Source: CAD feature listing. Evaluate the final solid. Frame: model axes, mm. Coordinates: 2 decimals unless noted, no trailing zeros. Write each loop counter-clockwise with the first axis right and the second up, starting at its lowest first coordinate (ties: lowest second). Pieces come first, ordered by that corner, then holes. Notation, with made-up numbers: M 66.25,42 L 125.25,42 A28 ccw 125.25,65 Z; hole C 27,34 d6. An arc over 180 degrees is marked long. Answer as CSV lines item,"result". Start each with the question number.
1. Line query: probe 1 along X at (y, z) = (8.5, -0.25); probe 2 along X at (y, z) = (-15, -0.4); probe 3 along X at (y, z) = (0, -0.25). Output: solid intervals per line, ascending. Write a range as [from, to].
2. Contact query for a flat-ended pin moving along its axis: pin 1 Ø3 at (x, y) = (26.5, -15) entering from +Z. Output: stop coordinate, or through.
3. Section C-C on y = 15. Return the cut outline in (x, z).
4. Section D-D on x = -4.25. Return the cut outline in (y, z).
5. Section A-A on y = 0. Return the cut outline in (x, z).
6. Section B-B on x = 26.5. Return the cut outline in (y, z), plus the area to 3 significant figures.
Autodesk Inventor part; units mm, degrees
ref_plane "YZ Plane" through (0, 0, 0) normal (1, 0, 0) x (0, 1, 0)
ref_plane "XZ Plane" through (0, 0, 0) normal (0, 1, 0) x (-1, 0, 0)
ref_plane "XY Plane" through (0, 0, 0) normal (0, 0, 1) x (1, 0, 0)
sketch "Sketch1" plane through (0, 0, 0) normal (0, 0, 1) x (1, 0, 0)
  line L0 (0, -42.5799) -> (0, 42.5799)
  line L1 (-42.5799, 0) -> (42.5799, 0)
  line L2 (-28, 30) -> (28, 30)
  line L3 (30, 28) -> (30, -28)
  line L4 (28, -30) -> (-28, -30)
  line L5 (-30, -28) -> (-30, 28)
  arc A0 (-28, 30) -> (-30, 28) centre (-28, 28) ccw
  arc A1 (30, 28) -> (28, 30) centre (28, 28) ccw
  arc A2 (28, -30) -> (30, -28) centre (28, -28) ccw
  arc A3 (-30, -28) -> (-28, -30) centre (-28, -28) ccw
  point P0 (0, 0)
  point P1 (-30, 30)
  point P2 (30, 30)
  point P3 (-22.4506, 22.4506)
  point P4 (-26.5, 15)
  point P5 (-15, 26.5)
  point P6 (-15, -26.5)
  point P7 (-22.4506, -22.4506)
  point P8 (-26.5, -15)
  point P9 (26.5, -15)
  point P10 (22.4506, -22.4506)
  point P11 (15, -26.5)
  point P12 (15, 26.5)
  point P13 (22.4506, 22.4506)
  point P14 (26.5, 15)
  point P15 (-21, 0)
  point P16 (21, 0)
  point P17 (-4.25, 0)
  point P18 (4.25, 0)
  point P19 (-23.5, 8.5)
  point P20 (-23.5, -8.5)
  point P21 (23.5, 8.5)
  point P22 (23.5, -8.5)
  dimension "d0" = 60
  dimension "d1" = 2
  dimension "d2" = 22.4506
  dimension "d3" = 22.4506
  dimension "d4" = 15
  dimension "d5" = 15
  dimension "d6" = 3.5
  dimension "d7" = 3.5
  dimension "d10" = 360
  dimension "d28" = 9
  dimension "d36" = 25.75
  dimension "d48" = 19.25
  dimension "d49" = 8.5
extrude "Extrusion1" add sketch "Sketch1" against normal blind 1.5
hole "Hole1" at (-22.4506, 22.4506, 0) at (22.4506, 22.4506, 0) at (22.4506, -22.4506, 0) at (-22.4506, -22.4506, 0) direction (0, 0, -1) diameter 3.4 end through all
hole "Hole2" at (-26.5, 15, 0) at (-15, 26.5, 0) at (-15, -26.5, 0) at (-26.5, -15, 0) at (26.5, -15, 0) at (15, -26.5, 0) at (15, 26.5, 0) at (26.5, 15, 0) direction (0, 0, -1) diameter 2.4 end through all
hole "Hole3" at (-21, 0, 0) at (21, 0, 0) direction (0, 0, -1) diameter 3 end through all
hole "Hole4" at (-4.25, 0, 0) at (4.25, 0, 0) at (-23.5, -8.5, 0) at (-23.5, 8.5, 0) at (23.5, 8.5, 0) at (23.5, -8.5, 0) direction (0, 0, -1) diameter 3 end through all
equation "\"encoder_axis\" = 8"
equation "\"encoder_emboss\" = 0"
equation "\"encoders\" = 0"
equation "\"encoder_width\" = 27"
equation "\"front_plate_thickness\" = 2"
equation "\"glass_thickness\" = 2"
equation "\"screw_distance_outside\" = 3.5"
equation "\"encoder_rad\" = 49"
equation "\"encoder_extrude_hight\" = 3"
equation "\"screw_distance_center\" = 15"
equation "\"ring_top_thickness\" = 2"
equation "\"ring_outer_bevel_depth\" = 0.5"
equation "\"ring_depth\" = 6"
equation "\"ring_outer_bevel_height\" = 3"
equation "\"ring_inner_bevel_depth\" = 3.5"
equation "\"ring_thickness\" = 9"
equation "\"hole_from_center\" = 63.5"
equation "\"circle_dimension_inner\" = 47"
equation "\"circle_dimension\" = 56"
equation "\"backplate_width\" = 60"
equation "\"hole_distance\" = 22.45064"
properties part number "pcb_board" material "ABS Plastic"
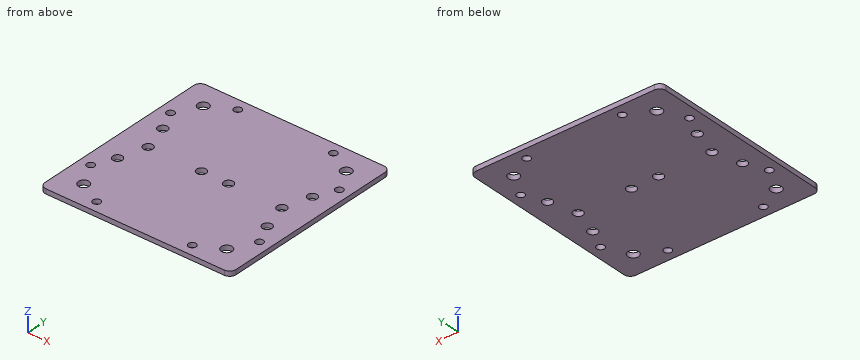
Values:
1,probe 1,"[-30, -25], [-22, 22], [25, 30]"
1,probe 2,"[-30, -27.7], [-25.3, 25.3], [27.7, 30]"
1,probe 3,"[-30, -22.5], [-19.5, -5.75], [-2.75, 2.75], [5.75, 19.5], [22.5, 30]"
2,pin 1,"z = 0"
3,outline,"M -30,-1.5 L -27.7,-1.5 L -27.7,0 L -30,0 Z; M -25.3,-1.5 L 25.3,-1.5 L 25.3,0 L -25.3,0 Z; M 27.7,-1.5 L 30,-1.5 L 30,0 L 27.7,0 Z"
4,outline,"M -30,-1.5 L -1.5,-1.5 L -1.5,0 L -30,0 Z; M 1.5,-1.5 L 30,-1.5 L 30,0 L 1.5,0 Z"
5,outline,"M -30,-1.5 L -22.5,-1.5 L -22.5,0 L -30,0 Z; M -19.5,-1.5 L -5.75,-1.5 L -5.75,0 L -19.5,0 Z; M -2.75,-1.5 L 2.75,-1.5 L 2.75,0 L -2.75,0 Z; M 5.75,-1.5 L 19.5,-1.5 L 19.5,0 L 5.75,0 Z; M 22.5,-1.5 L 30,-1.5 L 30,0 L 22.5,0 Z"
6,outline,"M -30,-1.5 L -16.2,-1.5 L -16.2,0 L -30,0 Z; M -13.8,-1.5 L 13.8,-1.5 L 13.8,0 L -13.8,0 Z; M 16.2,-1.5 L 30,-1.5 L 30,0 L 16.2,0 Z"
6,area,"82.8 mm²"
